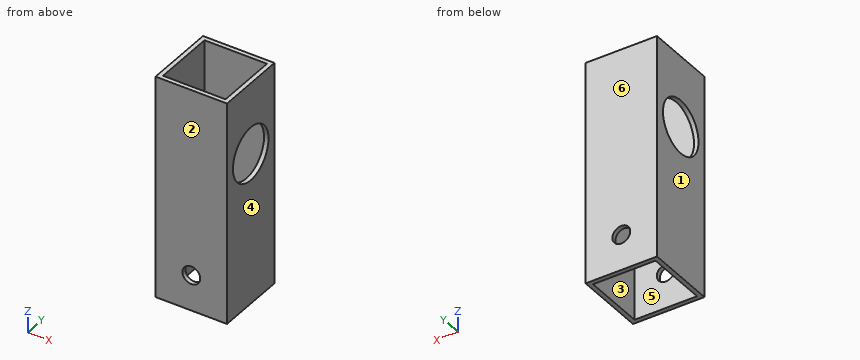
Autodesk Inventor part; units mm, degrees
ref_plane "YZ Plane" through (0, 0, 0) normal (1, 0, 0) x (0, 1, 0)
ref_plane "XZ Plane" through (0, 0, 0) normal (0, 1, 0) x (-1, 0, 0)
ref_plane "XY Plane" through (0, 0, 0) normal (0, 0, 1) x (1, 0, 0)
sketch "Sketch1" plane through (0, 0, 0) normal (0, 0, 1) x (1, 0, 0)
  line L0 (-11.051, 11.5151) -> (11.174, 11.5151)
  line L1 (11.174, 11.5151) -> (11.174, -10.7099)
  line L2 (11.174, -10.7099) -> (-11.051, -10.7099)
  line L3 (-11.051, -10.7099) -> (-11.051, 11.5151)
  line L4 (-12.6385, 13.1026) -> (12.7615, 13.1026)
  line L5 (12.7615, 13.1026) -> (12.7615, -12.2974)
  line L6 (12.7615, -12.2974) -> (-12.6385, -12.2974)
  line L7 (-12.6385, -12.2974) -> (-12.6385, 13.1026)
  point P0 (0, 0)
  dimension "d0" = 25.4
  dimension "d1" = 25.4
  dimension "d2" = 1.5875
  dimension "d3" = 1.5875
  dimension "d4" = 1.5875
  dimension "d5" = 1.5875
extrude "Extrusion1" add sketch "Sketch1" along normal blind 79.375
sketch "Sketch2" plane through (12.7615, -12.2974, 0) normal (1, 0, 0) x (0, 0, -1)
  circle A0 centre (-53.975, 12.7) radius 9.525
  line L0 (0, 0) -> (-79.375, 0)
  line L1 (-79.375, 0) -> (-79.375, 25.4)
  circle A1 centre (-33.655, 12.7) radius 3.175
  circle A2 centre (-74.295, 12.7) radius 3.175
  point P0 (0, 12.2974)
  dimension "d8" = 19.05
  dimension "d11" = 12.7
  dimension "d12" = 25.4
  dimension "d13" = 20.32
  dimension "d14" = 6.35
  dimension "d15" = 6.35
  dimension "d16" = 20.32
extrude "Extrusion2" cut sketch "Sketch2" against normal through all contours A0
sketch "Sketch3" plane through (-12.6385, 13.1026, 0) normal (0, 1, 0) x (1, 0, 0)
  circle A0 centre (12.7, -12.7) radius 3.175
  line L0 (0, 0) -> (0, -79.375)
  line L1 (25.4, 0) -> (0, 0)
  point P0 (12.6385, 0)
  dimension "d17" = 6.35
  dimension "d18" = 12.7
  dimension "d19" = 12.7
extrude "Extrusion3" cut sketch "Sketch3" against normal through all
equation "\"d3\" = d2"
equation "\"d4\" = d2"
equation "\"d5\" = d2"
equation "\"d16\" = d13"
properties part number "Diff Side Bar"
Source: CAD feature listing. Evaluate the final solid. Frame: model axes, mm. Face numbers are marked on the shaded views. A direction names the side the tool comes from. Coordinates: 2 decimals unless noted, no trailing zeros. Order: outer loops, then holes, each group sorted by start corner. A loop starts at its lowest first (then second) coordinate and runs counter-clockwise, first axis right, second up. Notation, with made-up numbers: (-28.5, -25.5) - (18.5, -25.5) arc R25 cw to (18.5, -12.5) - close; hole circle Ø5 at (75, 22). An arc over 180 degrees is marked (long way). One line per item, written item: value.
1) Reachability of the marked faces 5 and 6 from +Z, -Z, +X, -X, +Y, -Y: full face, straight path, thin tool, end or side. Return the list, or none.
Computed values:
face 5: +Z, -Z
face 6: +Z, -Z, +X, -X, +Y
2) Ray query, line 1 (X direction, y = 6, z = 72.5); line 2 (Y direction, x = -4.5, z = 53); line 3 (X direction, y = -11.15, z = 12.7). Return the intervals inside material, ascending. Write a range as [from, to].
Computed values:
line 1: x = [-12.64, -11.05], [11.17, 12.76]
line 2: y = [-12.3, -10.71], [11.52, 13.1]
line 3: x = [-12.64, -3.11], [3.24, 12.76]
3) Mould query, pull axis X, two halves, no side actions, for the marked faces 1, 2, 3 and 4. Classes: released by +X, released by -X, zero draft, split by the parting line, or undercut.
Computed values:
face 1: released by -X
face 2: zero draft
face 3: undercut
face 4: released by +X
4) Cut plane C-C on z = 12.7. Output: boundary loops of the cut face in (x, y).
Computed values:
outline: (-12.64, -12.3) - (-3.11, -12.3) - (-3.11, -10.71) - (-11.05, -10.71) - (-11.05, 11.52) - (-3.11, 11.52) - (-3.11, 13.1) - (-12.64, 13.1) - close; (3.24, -12.3) - (12.76, -12.3) - (12.76, 13.1) - (3.24, 13.1) - (3.24, 11.52) - (11.17, 11.52) - (11.17, -10.71) - (3.24, -10.71) - close
5) Cut plane D-D on x = 2.5. Output: boundary loops of the cut face in (y, z) (3 decimals).
Computed values:
outline: (-12.297, 0) - (-10.71, 0) - (-10.71, 10.667) - (-12.297, 10.667) - close; (-12.297, 14.733) - (-10.71, 14.733) - (-10.71, 79.375) - (-12.297, 79.375) - close; (11.515, 0) - (13.103, 0) - (13.103, 10.667) - (11.515, 10.667) - close; (11.515, 14.733) - (13.103, 14.733) - (13.103, 79.375) - (11.515, 79.375) - close
6) Cut plane A-A on z = 39.5. Output: boundary loops of the cut face in (x, y), plus the area to 3 significant figures.
Computed values:
outline: (-12.64, -12.3) - (12.76, -12.3) - (12.76, 13.1) - (-12.64, 13.1) - close; hole (-11.05, -10.71) - (11.17, -10.71) - (11.17, 11.52) - (-11.05, 11.52) - close
area: 151 mm^2
7) Cut plane B-B on x = -4.25. Output: boundary loops of the cut face in (y, z) (3 decimals), plus the area to 3 significant figures.
Computed values:
outline: (-12.297, 0) - (-10.71, 0) - (-10.71, 79.375) - (-12.297, 79.375) - close; (11.515, 0) - (13.103, 0) - (13.103, 79.375) - (11.515, 79.375) - close
area: 252 mm^2
